The drawing under review shows one solid part. Ordinate dimensions are in mm from its lowest x, y, z. A direction names the side the tool comes from. Coordinates: 2 decimals unless noted, no trailing zeros. Order: outer loops, then holes, each group sorted by start corner. A loop starts at its lowest first (then second) coordinate and runs counter-clockwise, first axis right, second up.
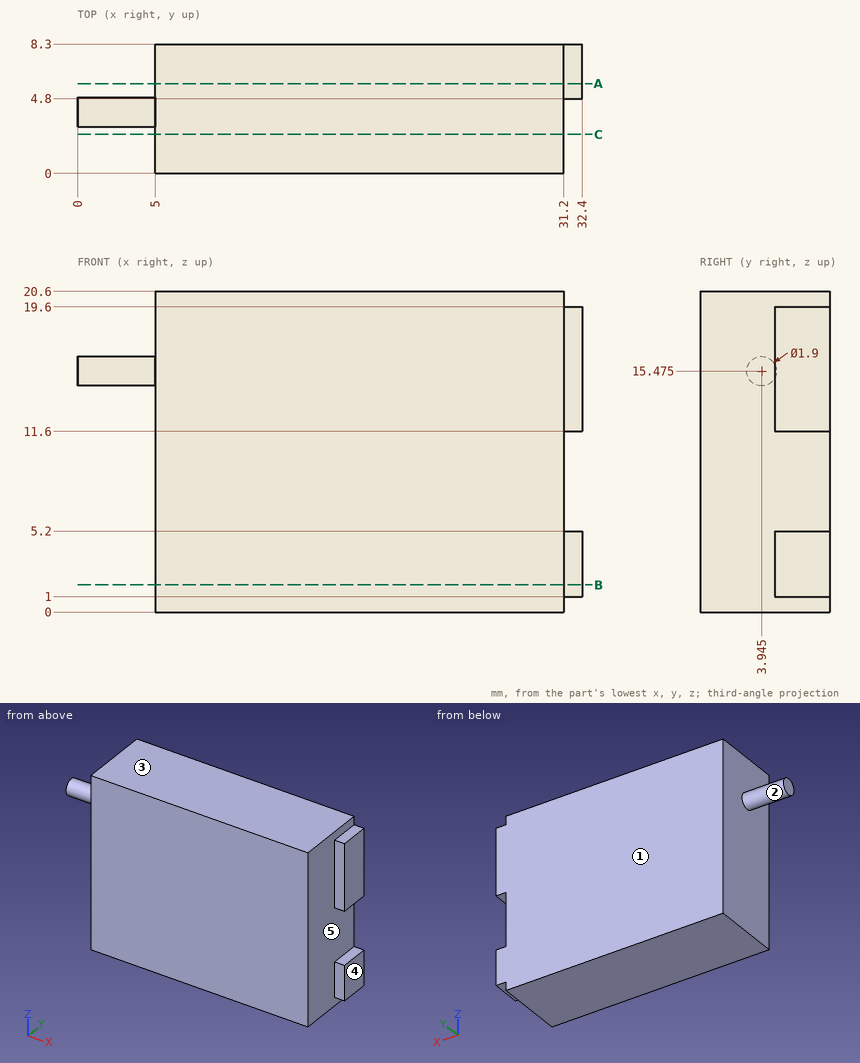
1. The part is to be moulded in two halves that separate along Z. For the marked faces 3, 4 and 5, say which applies: +Z half, -Z half, draft (parallel to the pull), parting line (faces both ways), or undercut.
Answer below:
face 3: +Z half
face 4: draft
face 5: undercut
2. Take a section at A-A, the plane y = 5.75. Give the boundary of the cut face in (x, z).
Answer below:
outline: (5, 0) - (31.2, 0) - (31.2, 1) - (32.4, 1) - (32.4, 5.2) - (31.2, 5.2) - (31.2, 11.6) - (32.4, 11.6) - (32.4, 19.6) - (31.2, 19.6) - (31.2, 20.6) - (5, 20.6) - close
3. To check wall thickness, follow L1, parallel to X at y = 0.5, z = 5; L2, parallel to X at y = 7, z = 16. State the ranges of each line that lie inside material, in increasing order.
Answer below:
L1: x = 5 to 31.2
L2: x = 5 to 32.4
4. Take a section at B-B, the plane z = 1.75. Give the boundary of the cut face in (x, y).
Answer below:
outline: (5, 0) - (31.2, 0) - (31.2, 4.8) - (32.4, 4.8) - (32.4, 8.3) - (5, 8.3) - close
5. Machinability: for the marked faces 1 and 2, which of the approach directions +Z, -Z, +X, -X, +Y, -Y give a long, thin tool a straight path to every point of the face, cutting with its end or side? Answer none if there is none.
Answer below:
face 1: +Z, -Z, +X, -X, +Y
face 2: -X
6. Clearance check with flat-ended pins moving along their axes: pin 1 Ø1.5 at (x, z) = (28, 11) entering from -Y; pin 2 Ø4 at (y, z) = (4.5, 10.5) entering from -X; pin 3 Ø1.3 at (x, y) = (32, 6.5) entering from -Z. State where each tip first meets the part, or that it passes through.
Answer below:
pin 1: stops at y = 0
pin 2: stops at x = 5
pin 3: stops at z = 1
7. Take a section at C-C, the plane y = 2.5. Give the boundary of the cut face in (x, z), plus the area to 3 significant figures.
Answer below:
outline: (5, 0) - (31.2, 0) - (31.2, 20.6) - (5, 20.6) - close
area: 540 mm2
